Design review of the part built by this model. Coordinates are the model's own, in mm. A direction names the side the tool comes from. Give positions to 0.01 mm unless a question says otherwise; leave off trailing zeros. Loops run counter-clockwise (first coordinate to the right, second up) from the corner with the lowest first, then second, coordinate; pieces in that order, holes last. Notation, with made-up numbers: (72.5, 4.5) -> (106.5, 4.5) arc R23 cw to (106.5, 31.5) -> close; hole circle Ø8 at (42.25, 42). An arc over 180 degrees is marked (long way). Answer as CSV lines item,"result".
from build123d import *

# Parameters (mm, degrees)
F0_R     = 1.5
F1_DEPTH = 3


with BuildPart() as f1:
    # F0 (on Top) → F1 (new body)
    with BuildSketch(Plane.XY):
        with BuildLine():
            ThreePointArc((6, -1), (6.292893, -0.292893), (7, 0))
            Line((7, 0), (97, 0))
            ThreePointArc((97, 0), (97.707107, 0.292893), (98, 1))
            Line((98, 1), (98, 3))
            ThreePointArc((98, 3), (97.12132, 5.12132), (95, 6))
            Line((95, 6), (3, 6))
            ThreePointArc((3, 6), (0.87868, 5.12132), (0, 3))
            Line((0, 3), (0, 1))
            Line((0, 1), (0, 0))
            Line((0, 0), (0, -61))
            ThreePointArc((0, -61), (0.87868, -63.12132), (3, -64))
            Line((3, -64), (5, -64))
            ThreePointArc((5, -64), (5.707107, -63.707107), (6, -63))
            Line((6, -63), (6, -1))
        make_face()
        with Locations((3, -61)):
            Circle(F0_R, mode=Mode.SUBTRACT)
        with Locations((3, 3)):
            Circle(F0_R, mode=Mode.SUBTRACT)
        with Locations((95, 3)):
            Circle(F0_R, mode=Mode.SUBTRACT)
    extrude(amount=F1_DEPTH)


solid = f1.part
Q1. We need section B-B, the plane x = 79. State the section outline as (y, z) points, and give its area (3 significant figures).
Filled sheet:
outline,"(0, 0) -> (6, 0) -> (6, 3) -> (0, 3) -> close"
area,"18.0 mm^2"
Q2. We need section A-A, the plane z = 1.85. State the section outline as (x, y) points.
Filled sheet:
outline,"(0, -61) arc R3 ccw to (3, -64) -> (5, -64) arc R1 ccw to (6, -63) -> (6, -1) arc R1 cw to (7, 0) -> (97, 0) arc R1 ccw to (98, 1) -> (98, 3) arc R3 ccw to (95, 6) -> (3, 6) arc R3 ccw to (0, 3) -> close; hole circle Ø3 at (3, -61); hole circle Ø3 at (3, 3); hole circle Ø3 at (95, 3)"
Q3. For faces 4 (the flat face through (51, 0, 1)), 5 (the flat face through (4, -64, 1)), list the 3-axis set-ups (+Z, -Z, +X, -X, +Y, -Y) from which the entire face can be reached by the end or side of a thin tool; tool diameter is ignored.
Filled sheet:
face 4,"+Z, -Z, +X, -Y"
face 5,"+Z, -Z, +X, -X, -Y"
Q4. Clearance check with a flat-ended pin moving along its axis: pin 1 Ø1.5 at (x, z) = (71.5, 2.5) entering from -Y. State where the tip first meets the part, or that it passes through.
Filled sheet:
pin 1,"stops at y = 0"
Q5. The part is to be moulded in two halves that separate along X. For faces 1 (the cylindrical face through (96.43, 3.45, 1.48)), 2 (the flat face through (27, 2, 3)), 3 (the cylindrical face through (0.9, 5.14, 1.48)), say which applies: pulls with the +X half, pulls with the -X half, needs draft (parallel to the pull), parting line crosses it, or undercut.
Filled sheet:
face 1,"undercut"
face 2,"needs draft"
face 3,"pulls with the -X half"
Q6. To check wall thickness, follow probe 1 along Y at (x, z) = (3, 1.25); probe 2 along Y at (x, z) = (95, 1.25); probe 3 along Y at (x, z) = (79, 2.65). State the ranges of each line that lie inside material, in increasing order. Write a range as from..to.
Filled sheet:
probe 1,"y = -64..-62.5, -59.5..1.5, 4.5..6"
probe 2,"y = 0..1.5, 4.5..6"
probe 3,"y = 0..6"
